Could you check a few things on this model? Use its own coordinates, in mm. Give positions to 0.01 mm unless a question says otherwise; leave off trailing zeros. Order: outer loops, then holes, each group sorted by start corner. A loop starts at its lowest first (then second) coordinate and runs counter-clockwise, first axis right, second up. Notation, with made-up numbers: (18.25, 45.25) -> (24.25, 45.25) arc R7 ccw to (24.25, 51.25) -> close; hole circle Ø3 at (58, 84). An arc over 180 degrees is marked (long way). Use one line per item in the form item = value. Start each with the question number.
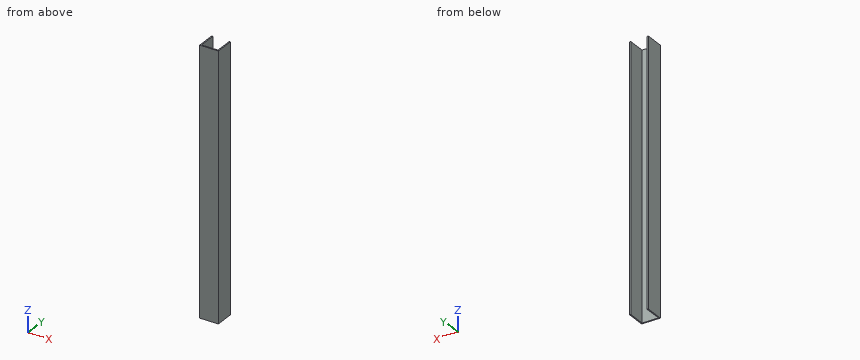
Autodesk Inventor part; units mm, degrees
ref_plane "YZ Plane" through (0, 0, 0) normal (1, 0, 0) x (0, 1, 0)
ref_plane "XZ Plane" through (0, 0, 0) normal (0, 1, 0) x (-1, 0, 0)
ref_plane "XY Plane" through (0, 0, 0) normal (0, 0, 1) x (1, 0, 0)
sketch "Sketch1" plane through (0, 0, 0) normal (0, 0, 1) x (1, 0, 0)
  line L0 (2.0066, 32.004) -> (0, 32.004)
  line L1 (0, 32.004) -> (0, 0)
  line L2 (0, 0) -> (2.0066, 0)
  line L3 (2.0066, 2.0066) -> (2.0066, 32.004)
  line L4 (2.0066, 0) -> (29.9974, 0)
  line L5 (29.9974, 2.0066) -> (2.0066, 2.0066)
  line L6 (29.9974, 0) -> (32.004, 0)
  line L7 (32.004, 0) -> (32.004, 32.004)
  line L8 (32.004, 32.004) -> (29.9974, 32.004)
  line L9 (29.9974, 32.004) -> (29.9974, 2.0066)
  dimension "d2" = 2.0066
  dimension "d3" = 32.004
sketch "Sketch2" plane through (0, 0, 0) normal (0, 0, 1) x (1, 0, 0)
  point P0 (0, 0)
extrude "Extrusion1" add sketch "Sketch1" along normal blind 450.85
properties part number "USEsolid7"
(1) Imagine slicing it at B-B (z = 103.5). Write out the boundary of the cut face in (x, y).
(2) I'm going to push a flat-ended pin straight in: pin 1 Ø15 at (y, z) = (15.5, 302.5) entering from -X. Where does the tip first touch, or does it pass through?
(3) Please list where these lines run through material, in increasing order: probe 1 along X at (y, z) = (10, 417); probe 2 along Y at (x, z) = (11.5, 225.5).
(4) Imagine slicing it at A-A (y = 9). Write out the boundary of the cut face in (x, z), plus the area to 3 significant figures.
(5) Imagine slicing it at C-C (x = 21.5). Write out the boundary of the cut face in (y, z), plus the area to 3 significant figures.
Calculated:
q1.outline = (0, 0) -> (32, 0) -> (32, 32) -> (30, 32) -> (30, 2.01) -> (2.01, 2.01) -> (2.01, 32) -> (0, 32) -> close
q2.pin_1 = 0
q3.probe_1 = 0 to 2.01, 30 to 32
q3.probe_2 = 0 to 2.01
q4.outline = (0, 0) -> (2.01, 0) -> (2.01, 450.85) -> (0, 450.85) -> close; (30, 0) -> (32, 0) -> (32, 450.85) -> (30, 450.85) -> close
q4.area = 1,810 mm2
q5.outline = (0, 0) -> (2.01, 0) -> (2.01, 450.85) -> (0, 450.85) -> close
q5.area = 905 mm2
